from build123d import *

# Parameters (mm, degrees)
AUFSATZ_LINEAR_AUSTRAGEN1_DEPTH = 35
SKIZZE3_R                       = 6
AUFSATZ_LINEAR_AUSTRAGEN2_DEPTH = 5
SKIZZE4_R                       = 6.5
AUFSATZ_LINEAR_AUSTRAGEN3_DEPTH = 0.1
SKIZZE9_R                       = 1.7
AUFSATZ_LINEAR_AUSTRAGEN4_DEPTH = 4


with BuildPart() as part:
    # Skizze1 → Aufsatz-Linear austragen1 (new body)
    with BuildSketch(Plane(origin=(0, 0, 0), x_dir=(0, 0, -1), z_dir=(1, 0, 0))):
        Polygon((0, 0), (11.970705016, 0), (26.82, 0), (26.82, 154.689241728), (11.970705016, 154.689241728), (0, 121.8), align=None)
    extrude(amount=AUFSATZ_LINEAR_AUSTRAGEN1_DEPTH)

    # Skizze3 → Aufsatz-Linear austragen2 (add)
    with BuildSketch(Plane(origin=(0, 14.247893414, 39.14576543), x_dir=(1, 0, 0), z_dir=(0, 0.342020143, 0.939692621))):
        with Locations((17.5, 131.954561212)):
            Circle(SKIZZE3_R)
    extrude(amount=AUFSATZ_LINEAR_AUSTRAGEN2_DEPTH)

    # Skizze4 → Aufsatz-Linear austragen3 (add)
    with BuildSketch(Plane(origin=(0, 14.247893414, 39.14576543), x_dir=(1, 0, 0), z_dir=(0, 0.342020143, 0.939692621))):
        with Locations((17.5, 131.954561212)):
            Circle(SKIZZE4_R)
    extrude(amount=AUFSATZ_LINEAR_AUSTRAGEN3_DEPTH)

    # Skizze9 → Aufsatz-Linear austragen4 (add)
    with BuildSketch(Plane.XZ):
        Polygon((35, -26.82), (50, -14.233505532), (50, 12.586494468), (35, 0), align=None)
        with Locations((46, 4.008466786)):
            Circle(SKIZZE9_R, mode=Mode.SUBTRACT)
        with Locations((39, -18.241972318)):
            Circle(SKIZZE9_R, mode=Mode.SUBTRACT)
        Polygon((0, 0), (0, -26.82), (-15, -14.233505532), (-15, 12.586494468), align=None)
        with Locations((-4, -18.241972318)):
            Circle(SKIZZE9_R, mode=Mode.SUBTRACT)
        with Locations((-11, 4.008466786)):
            Circle(SKIZZE9_R, mode=Mode.SUBTRACT)
    extrude(amount=-AUFSATZ_LINEAR_AUSTRAGEN4_DEPTH)


solid = part.part
Geometry check sheet. Reference: the model listing, model coordinates, mm. A direction names the side the tool comes from. Round coordinates to 2 decimals unless told otherwise and drop trailing zeros. Loops run counter-clockwise (first coordinate to the right, second up) from the corner with the lowest first, then second, coordinate; pieces in that order, holes last. Notation, with made-up numbers: (-10.5, -36.5) -> (28.5, -36.5) arc R11 cw to (28.5, -27.5) -> close; hole circle Ø10 at (17, 37). An arc over 180 degrees is marked (long way). Answer as a JSON object with one key per item and string values. Group by question number.
Item 1: Cross-section at C-C, the plane z = -10. Record the cut outline in (x, y), plus the area to 3 significant figures.
Item 2: Cross-section at D-D, the plane y = 115. Record the cut outline in (x, z).
Item 3: Depth check by flat-ended pin: pin 1 Ø13.5 at (y, z) = (83, -12) entering from -X; pin 2 Ø21.5 at (y, z) = (102.5, -18.5) entering from +X; pin 3 Ø2 at (x, y) = (23, 24) entering from +Z. Enter the tip coordinate at first touch or a pass-through.
Item 4: Cross-section at A-A, the plane z = 10. Record the cut outline in (x, y).
Item 5: Release check for a two-part mould opening along Z. For faces 5 (the face through (38.63, 1.97, -19.9)), 6 (the face through (42.605, 1.972, 6.381)), 7 (the face through (17, 0, -11)) record: pulls with the +Z half, pulls with the -Z half, needs draft (parallel to the pull), parting line crosses it, or undercut.
Item 6: Cross-section at B-B, the plane x = -4. Record the cut outline in (y, z).
Item 7: Thickness scan on line 1 along X through (y, z) = (63, -5); line 2 along Y through (x, z) = (38.5, -1.5); line 3 along Z through (x, y) = (4, 92). Record the ranges inside material, lowest first.
Item 8: Set-up check for faces 1 (the face through (42, 4, -7)), 2 (the face through (42.4, 1.97, -20.61)), 3 (the face through (-7.605, 1.972, 6.381)), 4 (the face through (0, 80, -13)): record each of +Z, -Z, +X, -X, +Y, -Y from which the full face is reachable in a straight line by a thin tool's end or side.
Determined:
{
 "1": {"outline": "(-15, 0) -> (50, 0) -> (50, 4) -> (35, 4) -> (35, 149.27) -> (0, 149.27) -> (0, 4) -> (-15, 4) -> close", "area": "5,340 mm²"},
 "2": {"outline": "(0, -26.82) -> (35, -26.82) -> (35, 0) -> (0, 0) -> close"},
 "3": {"pin 1": "stops at x = 0", "pin 2": "stops at x = 35", "pin 3": "stops at z = 0"},
 "4": {"outline": "(-15, 0) -> (-11.92, 0) -> (-11.92, 4) -> (-15, 4) -> close; (46.92, 0) -> (50, 0) -> (50, 4) -> (46.92, 4) -> close"},
 "5": {"face 5": "undercut", "face 6": "pulls with the +Z half", "face 7": "needs draft"},
 "6": {"outline": "(0, -23.46) -> (4, -23.46) -> (4, -19.94) -> (0, -19.94) -> close; (0, -16.54) -> (4, -16.54) -> (4, 3.36) -> (0, 3.36) -> close"},
 "7": {"line 1": "x = 0 to 35", "line 2": "y = 0 to 4", "line 3": "z = -26.82 to 0"},
 "8": {"face 1": "+Z, -Z, +X, +Y", "face 2": "-Z, +X, +Y, -Y", "face 3": "+Z, +Y, -Y", "face 4": "+Z, -Z, -X, +Y"}
}
